Part model, mm, in its own coordinate system. A direction names the side the tool comes from. Round coordinates to 2 decimals unless told otherwise and drop trailing zeros. Write each loop counter-clockwise with the first axis right and the second up, starting at its lowest first coordinate (ties: lowest second). Pieces come first, ordered by that corner, then holes.
Autodesk Inventor part; units mm, degrees
ref_plane "YZ Plane" through (0, 0, 0) normal (1, 0, 0) x (0, 1, 0)
ref_plane "XZ Plane" through (0, 0, 0) normal (0, 1, 0) x (-1, 0, 0)
ref_plane "XY Plane" through (0, 0, 0) normal (0, 0, 1) x (1, 0, 0)
sketch "Sketch1" plane through (0, 0, 0) normal (0, 0, 1) x (1, 0, 0)
  circle A0 centre (36.1481, 50.2593) radius 25
  circle A1 centre (36.1481, 50.2593) radius 19
  line L0 (36.1481, 75.2593) -> (1.1481, 75.2593)
  line L1 (36.1481, 85.2593) -> (-8.8519, 85.2593)
  line L2 (-8.8519, 85.2593) -> (-8.8519, 75.2593)
  line L3 (36.1481, 85.2593) -> (36.1481, 75.2593)
  line L4 (1.1481, 75.2593) -> (-8.8519, 75.2593)
  line L5 (36.1481, 25.2593) -> (1.1481, 25.2593)
  line L6 (36.1481, 15.2593) -> (-8.8519, 15.2593)
  line L7 (1.1481, 25.2593) -> (-8.8519, 25.2593)
  line L8 (36.1481, 15.2593) -> (36.1481, 25.2593)
  line L9 (-8.8519, 15.2593) -> (-8.8519, 25.2593)
  line L10 (36.1481, 85.2593) -> (53.6445, 68.1164)
  line L11 (36.1481, 15.2593) -> (53.6445, 32.4021)
  arc A2 (25.8947, 73.0598) -> (22.1511, 75.2593) centre (22.1511, 70.9735) ccw
  arc A3 (25.8027, 25.2593) -> (23.935, 28.4455) centre (22.1511, 25.2593) ccw
  point P0 (0, 0)
  dimension "d0" = 38
  dimension "d1" = 10
extrude "Extrusion1" add sketch "Sketch1" along normal blind 40
sketch "Sketch2" plane through (-8.8519, 15.2593, 0) normal (0, -1, 0) x (1, 0, 0)
  line L0 (0, 0) -> (0, 40)
  line L1 (0, 20) -> (12, 20)
  circle A0 centre (12, 20) radius 8
  point P0 (8.8519, 0)
  dimension "d4" = 12
  dimension "d5" = 16
extrude "Extrusion2" cut sketch "Sketch2" against normal blind 80
sketch "Sketch4" plane through (0, 0, 0) normal (1, 0, 0) x (0, 1, 0)
  line L0 (15.2593, 0) -> (15.2593, 40)
  line L1 (15.2593, 20) -> (85.6982, 20)
  point P0 (0, 0)
  point P1 (50.4787, 20)
hole "Hole1" at (0, 50.4787, 20) direction (1, 0, 0) diameter 4.917 depth 85.1 tip angle 118
properties part number "MANCAL_SUPORTE_EIXO" material "SAE 1010/1020"
Q1. Cut at C-C on x = 16. Write the cut outline in (y, z), plus the area to 3 significant figures.
Values follow:
outline: (15.26, 0) - (25.26, 0) - (25.26, 40) - (15.26, 40) - close; (35.46, 0) - (65.06, 0) - (65.06, 40) - (35.46, 40) - close; (75.26, 0) - (85.26, 0) - (85.26, 40) - (75.26, 40) - close; hole circle Ø4.92 at (50.48, 20)
area: 1,970 mm2
Q2. Wall check: L1, parallel to Y at x = 6, z = 7.5; L2, parallel to Y at x = 15.5, z = 20; L3, parallel to Y at x = 13.75, z = 20. Give the ranges that are in metal, low to high.
Values follow:
L1: y = 15.26 to 25.26, 75.26 to 85.26
L2: y = 15.26 to 25.26, 36.16 to 48.02, 52.94 to 64.35, 75.26 to 85.26
L3: y = 15.26 to 25.26, 39.15 to 48.02, 52.94 to 61.36, 75.26 to 85.26
Q3. Which spindle directions (+Z, -Z, +X, -X, +Y, -Y) get a long thin tool onto all of the face, cutting with end or side? Do faces 1 (the flat face through (13, 25.259, 20)), 2 (the flat face through (16, 48, 40)). Say none if no direction does.
Values follow:
face 1: +Z, -Z, -X
face 2: +Z, +X, -X, +Y, -Y
Q4. Cut at A-A on z = 16. Write the cut outline in (x, y) (1 decimal), plus the area to 3 significant figures.
Values follow:
outline: (-8.9, 15.3) - (-3.8, 15.3) - (-3.8, 25.3) - (-8.9, 25.3) - close; (-8.9, 75.3) - (-3.8, 75.3) - (-3.8, 85.3) - (-8.9, 85.3) - close; (10.1, 15.3) - (36.1, 15.3) - (53.6, 32.4) arc R25 ccw to (53.6, 68.1) - (36.1, 85.3) - (10.1, 85.3) - (10.1, 75.3) - (22.2, 75.3) arc R4.3 cw to (25.9, 73.1) arc R25 ccw to (23.9, 28.4) arc R3.7 cw to (25.8, 25.3) - (10.1, 25.3) - close; hole circle Ø38 at (36.1, 50.3)
area: 1,600 mm2
Q5. Cut at D-D on x = 0. Write the cut outline in (y, z), plus the area to 3 significant figures.
Values follow:
outline: (15.26, 0) - (25.26, 0) - (25.26, 12.65) - (15.26, 12.65) - close; (15.26, 27.35) - (25.26, 27.35) - (25.26, 40) - (15.26, 40) - close; (75.26, 0) - (85.26, 0) - (85.26, 12.65) - (75.26, 12.65) - close; (75.26, 27.35) - (85.26, 27.35) - (85.26, 40) - (75.26, 40) - close
area: 506 mm2
Q6. Mould opens along Y. For faces 3 (the flat face through (-8.852, 80, 20)), 4 (the cylindrical face through (54.27, 44.55, 19.72)), 5 (the cylindrical face through (58.097, 50.371, 17.544)), 6 (the flat face through (44.77, 76.81, 19.72)) say: +Y half, -Y half, draft (parallel to the pull), parting line (faces both ways), or undercut.
Values follow:
face 3: draft
face 4: undercut
face 5: undercut
face 6: +Y half
Q7. Cut at B-B on y = 51.5. Write the cut outline in (x, z).
Values follow:
outline: (11.18, 0) - (17.19, 0) - (17.19, 17.76) - (11.18, 17.76) - close; (11.18, 22.24) - (17.19, 22.24) - (17.19, 40) - (11.18, 40) - close; (55.11, 0) - (61.12, 0) - (61.12, 17.76) - (55.11, 17.76) - close; (55.11, 22.24) - (61.12, 22.24) - (61.12, 40) - (55.11, 40) - close
Q8. Drop flat-ended pins along their axis: pin 1 (3 mm diameter, centred on y = 45, z = 10.5, fed in from +X); pin 2 (10 mm diameter, centred on y = 47.5, z = 13.5, fed in from -X); pin 3 (1.5 mm diameter, centred on y = 28.5, z = 7.5, fed in from +X). Give the stop position or say it passes through.
Values follow:
pin 1: stops at x = 60.86
pin 2: stops at x = 11.15
pin 3: stops at x = 50.43
